Input: part model. Units: mm. Frame: model coordinates. A direction names the side the tool comes from. Round coordinates to 2 decimals unless told otherwise and drop trailing zeros. Loops run counter-clockwise (first coordinate to the right, second up) from the corner with the lowest first, then second, coordinate; pieces in that order, holes last. Notation, with made-up numbers: M -39.75,33.5 L -5.75,33.5 A37 cw -5.75,69.5 Z; hole C 45.5,-32 d2. An arc over 180 degrees is marked long. Put each result on its own line as item: value. Start each with the question number.
1) Pin query (flat end, axial travel): pin 1 (4 mm diameter, centred on x = 34, z = -4, fed in from +Y); pin 2 (8 mm diameter, centred on x = -22.5, y = 4.5, fed in from +Z); pin 3 (8 mm diameter, centred on x = 0, z = 0, fed in from -Y); pin 4 (8 mm diameter, centred on x = -26.5, z = -2, fed in from +Y). Return the tip coordinate at first contact, or that it passes through.
2) Reachability of faces 1 (the face through (-42.34, -0.867, 3.905)), 2 (the face through (-0.1, -5, 3.3)), 3 (the face through (-52.656, -3.796, -0.167)) from +Z, -Z, +X, -X, +Y, -Y: full face, straight path, thin tool, end or side. Return the list, or none.
3) Section B-B on x = -12.5. Output: boundary loops of the cut face in (y, z).
4) Section A-A on x = 0. Output: boundary loops of the cut face in (y, z).
5) Draft query along Z for faces 4 (the face through (-31.2, -4, -4)), 5 (the face through (1.532, 4.443, 4.864)), 6 (the face through (31.71, -1.08, 4.88)). Return one class per face: +Z half, -Z half, draft (parallel to the pull), parting line (faces both ways), or undercut.
6) Section C-C on y = 6.25. Output: boundary loops of the cut face in (x, z), plus the area to 3 significant figures.
7) Section D-D on z = -6. Output: boundary loops of the cut face in (x, y), plus the area to 3 significant figures.
8) Line query: probe 1 along X at (y, z) = (5.5, 0.25); probe 2 along X at (y, z) = (-1.35, 0); probe 3 along X at (y, z) = (3, -6.5). Output: solid intervals per line, ascending.
from build123d import *

# Parameters (mm, degrees)
SKETCH1_R               = 9
BOSS_EXTRUDE1_DEPTH     = 31.2
CUT_EXTRUDE1_DEPTH      = 34.696290597
CUT_EXTRUDE1_DEPTH_BACK = 34.696290597
SKETCH2_R               = 5.1
SKETCH7_R               = 5.25
SKETCH7_R_2             = 3
BOSS_EXTRUDE2_DEPTH     = 5


with BuildPart() as part:
    # Sketch1 → Boss-Extrude1 (new, symmetric)
    with BuildSketch(Plane(origin=(0, 0, 0), x_dir=(0, 0, -1), z_dir=(1, 0, 0))):
        Circle(SKETCH1_R)
    extrude(amount=BOSS_EXTRUDE1_DEPTH, both=True)

    # Sketch2 → Cut-Extrude1 (cut, two sides: drawn at the far end of the back side and taken through both)
    with BuildSketch(Plane(origin=(0, 0, 0), x_dir=(1, 0, 0), z_dir=(0, 1, 0)).offset(-CUT_EXTRUDE1_DEPTH_BACK)):
        with Locations(Location((0, 0, 0), (0, 0, 270))):
            Circle(SKETCH2_R)
    extrude(amount=CUT_EXTRUDE1_DEPTH + CUT_EXTRUDE1_DEPTH_BACK, mode=Mode.SUBTRACT)

    # Sketch6 → Revolve1 (revolve)
    with BuildSketch(Plane.XY):
        Polygon((31.2, 0), (31.2, 5), (32.2, 5), (32.2, 4), (52.2, 4), (52.2, 3.8), (53.1, 3.8), (53.1, 4), (54.1, 4), (54.1, 0), align=None)
    revolve1 = revolve(axis=Axis((54.1, 0, 0), (-1, 0, 0)))

    # Mirror1: Revolve1 across plane
    add(revolve1.mirror(Plane(origin=(0, 0, 0), x_dir=(0, 0, 1), z_dir=(1, 0, 0))))

    # Sketch7 → Boss-Extrude2 (add)
    with BuildSketch(Plane(origin=(0, 0, 0), x_dir=(1, 0, 0), z_dir=(0, 1, 0))):
        Circle(SKETCH7_R)
        with Locations(Location((0, 0, 0), (0, 0, 270))):
            Circle(SKETCH7_R_2, mode=Mode.SUBTRACT)
    extrude(amount=-BOSS_EXTRUDE2_DEPTH)


solid = part.part
Geometry results:
1. pin 1: stops at y = 3.9
1. pin 2: stops at z = 8.99
1. pin 3: stops at y = -5
1. pin 4: stops at y = 9
2. face 1: -X
2. face 2: -Y
2. face 3: none
3. outline: C 0,0 d18
4. outline: M -7.42,-5.1 A9 ccw 7.42,-5.1 L 0,-5.1 L 0,-3 L -5,-3 L -5,-5.1 Z; M -7.42,5.1 L -5,5.1 L -5,3 L 0,3 L 0,5.1 L 7.42,5.1 A9 ccw Z
5. face 4: draft
5. face 5: undercut
5. face 6: parting line
6. outline: M -31.2,-6.48 L 31.2,-6.48 L 31.2,6.48 L -31.2,6.48 Z; hole C 0,0 d10.2
6. area: 726 mm²
7. outline: M -31.2,-6.71 L 31.2,-6.71 L 31.2,6.71 L -31.2,6.71 Z
7. area: 837 mm²
8. probe 1: x = -31.2 to -5.09, 5.09 to 31.2
8. probe 2: x = -54.1 to -3, 3 to 54.1
8. probe 3: x = -31.2 to 31.2
